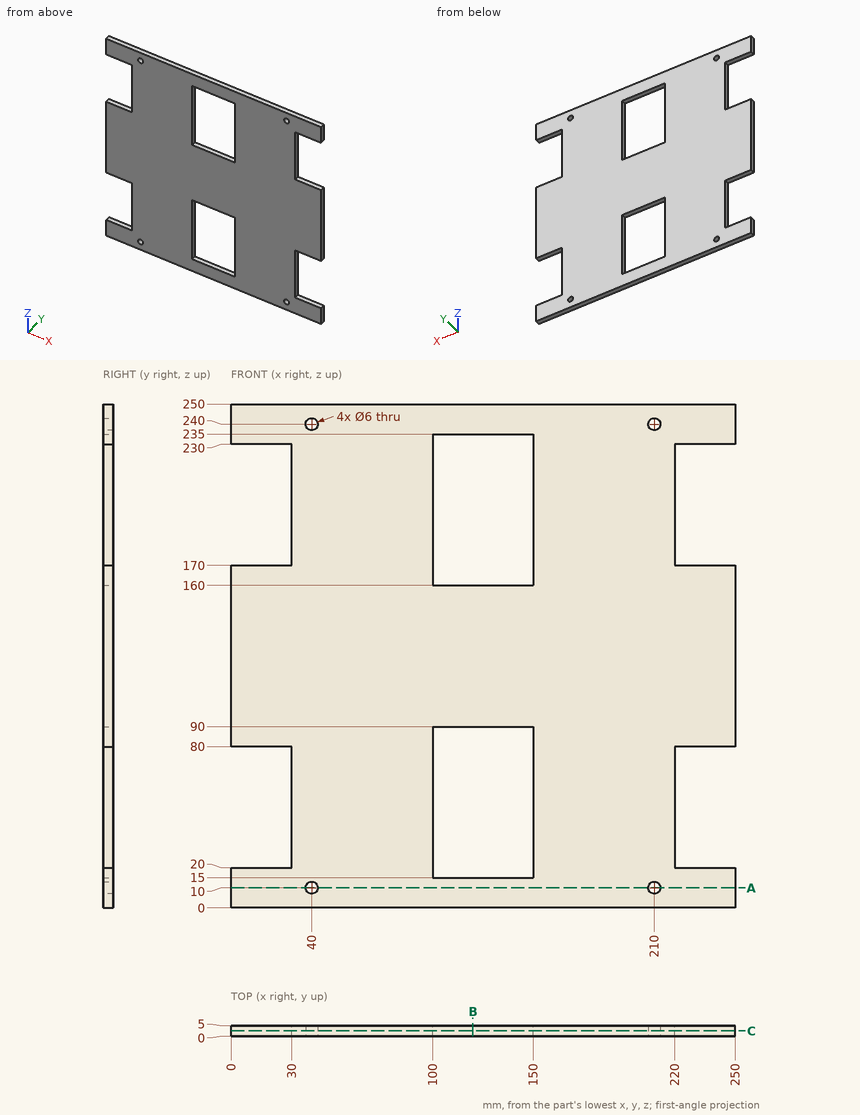
Study the drawing (mm; zero at the part's minimum x, y, z) and answer. Round coordinates to 2 decimals unless told otherwise and drop trailing zeros. Order: outer loops, then holes, each group sorted by start corner. A loop starts at its lowest first (then second) coordinate and runs counter-clockwise, first axis right, second up. Notation, with made-up numbers: M -40,75 L -12,75 A9 ccw -12,83 Z; hole C 53,35.5 d10. An arc over 180 degrees is marked long. One line per item, written item: value.
Q1. Straight lines are drawn through the part: line 1 (Z direction, x = 210, y = 2); line 2 (X direction, y = 3.2, z = 240); line 3 (X direction, y = 0.3, z = 227). For each, find the intervals that lie inside material, in ascending order.
Derived:
line 1: 0 to 7, 13 to 237, 243 to 250
line 2: 0 to 37, 43 to 207, 213 to 250
line 3: 30 to 100, 150 to 220
Q2. Find section A-A on z = 10. Write down the section's boundary in (x, y).
Derived:
outline: M 0,0 L 37,0 L 37,5 L 0,5 Z; M 43,0 L 207,0 L 207,5 L 43,5 Z; M 213,0 L 250,0 L 250,5 L 213,5 Z
Q3. Find section C-C on y = 2.55. Give the number of separate pieces and of enclosed holes in the cut face, then the cut area to 3 significant figures.
Derived:
separate pieces: 1
enclosed holes: 6
area: 47,700 mm²
Q4. A flat-ended cylindrical pin translates along its axis: pin 1 (1 mm diameter, centred on y = 1.5, z = 26, fed in from +X). Find the tip coordinate at first contact, or state that the pin passes through.
Derived:
pin 1: x = 220
Q5. Find section B-B on x = 120. Write down the section's boundary in (y, z), then the cut area to 3 significant figures.
Derived:
outline: M 0,0 L 5,0 L 5,15 L 0,15 Z; M 0,90 L 5,90 L 5,160 L 0,160 Z; M 0,235 L 5,235 L 5,250 L 0,250 Z
area: 500 mm²
